from build123d import *

# Parameters (mm, degrees)
F0_R     = 34.9158107131
F1_DEPTH = 152.4
F2_R     = 25
F3_R     = 25.7826386029
F4_DEPTH = 137.16
F5_DEPTH = 12.7
F6_SCALE = 0.9


with BuildPart() as f1:
    # F0 (on Top) → F1 (new body)
    with BuildSketch(Plane.XY):
        Circle(F0_R)
    extrude(amount=F1_DEPTH)

    # F2
    f2_edges = [f1.edges().sort_by_distance(p)[0] for p in [
        (-34.915811, 0, 152.4),
    ]]
    fillet(f2_edges, radius=F2_R)

    # F3 (on face) → F4 (cut)
    with BuildSketch(Plane(origin=(0, 0, 0), x_dir=(1, 0, 0), z_dir=(0, 0, -1))):
        Circle(F3_R)
    extrude(amount=-F4_DEPTH, mode=Mode.SUBTRACT)

    # F5 (cut): a face of the model
    f5_faces = [f1.faces().sort_by_distance(p)[0] for p in [
        (-33.9282424521, 0, 0),
    ]]
    extrude(f5_faces, amount=-F5_DEPTH, mode=Mode.SUBTRACT)


with BuildPart() as f1_1:
    # F6: moved
    add(f1.part.scale(F6_SCALE))


solid = f1_1.part
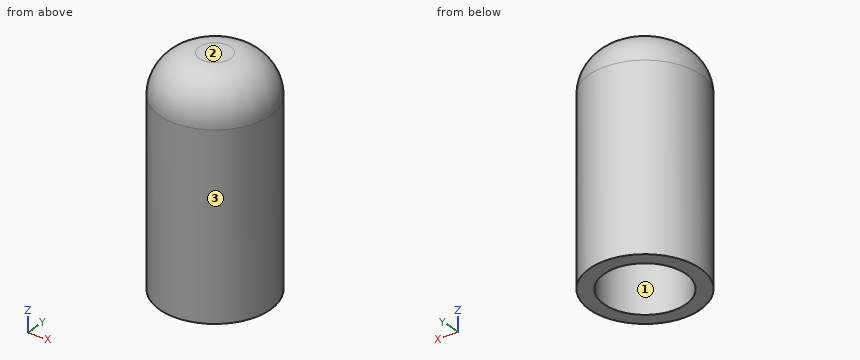
Work out the finished part from the listing and answer in its coordinate system (mm). Face numbers are marked on the shaded views. Give positions to 0.01 mm unless a question says otherwise; leave off trailing zeros. Loops run counter-clockwise (first coordinate to the right, second up) from the corner with the lowest first, then second, coordinate; pieces in that order, holes last. Notation, with made-up numbers: (25.25, 66.5) -> (78.25, 66.5) arc R16 cw to (78.25, 72.5) -> close; hole circle Ø2 at (-9.75, 1.5). An arc over 180 degrees is marked (long way). Use a Markdown table: item, result. Add a question column.
1. Flat-ended cylindrical pins translate along their axes: pin 1 Ø3 at (y, z) = (24.5, 59.5) entering from +X; pin 2 Ø1.5 at (y, z) = (-24.5, 34.5) entering from -X; pin 3 Ø4 at (x, y) = (-17, 9.5) entering from -Z. Find the tip coordinate at first contact, or state that the pin passes through.
2. Find the intervals of material crossed by probe 1 along Y at (x, z) = (0, 98.5); probe 2 along Y at (x, z) = (-2.5, 101), in increasing order.
3. Section A-A on z = 27.5 is taken. Determine the outline of the cut face in (x, y), and give its area (3 significant figures).
4. Determine the mould class of the marked faces 1, 2 and 3 for opening direction X: released by +X, released by -X, zero draft, split by the parting line, or undercut.
Results below:
| question | item | result |
|---|---|---|
| 1 | pin 1 | stops at x = 21.41 |
| 1 | pin 2 | stops at x = -20.58 |
| 1 | pin 3 | stops at z = 123.44 |
| 2 | probe 1 | y = -31.42 to -23.2, 23.2 to 31.42 |
| 2 | probe 2 | y = -31.32 to -23.07, 23.07 to 31.32 |
| 3 | outline | circle Ø62.85 at (0, 0); hole circle Ø46.41 at (0, 0) |
| 3 | area | 1,410 mm^2 |
| 4 | face 1 | undercut |
| 4 | face 2 | zero draft |
| 4 | face 3 | split by the parting line |
